```python
from build123d import *

# Parameters (mm, degrees)
SKETCH1_R           = 1.75
BOSS_EXTRUDE1_DEPTH = 1.6


with BuildPart() as part:
    # Sketch1 → Boss-Extrude1 (new body)
    with BuildSketch(Plane(origin=(0, 0, 0), x_dir=(1, 0, 0), z_dir=(0, 1, 0))):
        with BuildLine():
            Line((24.696313384, 21.403189927), (-19.414899465, 47.563680085))
            ThreePointArc((-19.414899465, 47.563680085), (-20.786874634, 49.384536896), (-20.482680557, 51.644028288))
            Line((-20.482680557, 51.644028288), (17.162414168, 116.847245007))
            ThreePointArc((17.162414168, 116.847245007), (19.546471274, 118.676596366), (22.525800971, 118.28436017))
            Line((22.525800971, 118.28436017), (70.987796177, 90.304814192))
            ThreePointArc((70.987796177, 90.304814192), (77.999004119, 90.304814192), (81.50460809, 96.376698381))
            Line((81.50460809, 96.376698381), (81.50460809, 182.02519482))
            ThreePointArc((81.50460809, 182.02519482), (80.873629228, 187.452491566), (79.01435205, 192.590270527))
            Line((79.01435205, 192.590270527), (69.144094326, 212.364639151))
            ThreePointArc((69.144094326, 212.364639151), (65.989183491, 217.196365343), (61.81193417, 221.177524531))
            Line((61.81193417, 221.177524531), (44.99314954, 233.854205885))
            Line((44.99314954, 233.854205885), (-23.199197227, 273.225075648))
            ThreePointArc((-23.199197227, 273.225075648), (-28.860512938, 273.225075648), (-31.691170793, 268.322232423))
            Line((-31.691170793, 268.322232423), (-31.691170793, 207.371759387))
            ThreePointArc((-31.691170793, 207.371759387), (-32.56985045, 205.250439044), (-34.691170793, 204.371759387))
            Line((-34.691170793, 204.371759387), (-106.595635326, 204.371759387))
            ThreePointArc((-106.595635326, 204.371759387), (-108.71695567, 205.250439044), (-109.595635326, 207.371759387))
            Line((-109.595635326, 207.371759387), (-109.595635326, 268.322232423))
            ThreePointArc((-109.595635326, 268.322232423), (-112.426293182, 273.225075648), (-118.087608892, 273.225075648))
            Line((-118.087608892, 273.225075648), (-186.279955659, 233.854205885))
            Line((-186.279955659, 233.854205885), (-204.21495553, 220.336208987))
            ThreePointArc((-204.21495553, 220.336208987), (-207.400637767, 217.300070339), (-209.806657286, 213.615266508))
            Line((-209.806657286, 213.615266508), (-217.247579174, 198.707901735))
            ThreePointArc((-217.247579174, 198.707901735), (-221.386722215, 187.270122423), (-222.791414209, 175.187815477))
            Line((-222.791414209, 175.187815477), (-222.791414209, 96.376698381))
            ThreePointArc((-222.791414209, 96.376698381), (-219.069332913, 89.929864467), (-211.625170321, 89.929864467))
            Line((-211.625170321, 89.929864467), (-163.512384372, 117.707794386))
            ThreePointArc((-163.512384372, 117.707794386), (-160.504762554, 118.10375531), (-158.098066116, 116.257032182))
            Line((-158.098066116, 116.257032182), (-120.496410943, 51.129054973))
            ThreePointArc((-120.496410943, 51.129054973), (-120.196709676, 48.852597838), (-121.594487155, 47.030978762))
            Line((-121.594487155, 47.030978762), (-165.983119503, 21.403189927))
            Line((-165.983119503, 21.403189927), (-174.676412504, 16.182853027))
            ThreePointArc((-174.676412504, 16.182853027), (-176.124776412, 13.818668342), (-175.016914475, 11.277060748))
            Line((-175.016914475, 11.277060748), (-168.860075369, 6.304549502))
            Line((-168.860075369, 6.304549502), (-141.286806119, 0))
            Line((-141.286806119, 0), (0, 0))
            Line((0, 0), (27.57326925, 6.304549502))
            Line((27.57326925, 6.304549502), (33.730108356, 11.277060748))
            ThreePointArc((33.730108356, 11.277060748), (34.837970293, 13.818668342), (33.389606385, 16.182853027))
            Line((33.389606385, 16.182853027), (24.696313384, 21.403189927))
        make_face()
        with Locations(Location((-123.091146174, 191.349343748, 0), (0, 0, 270))):
            Circle(SKETCH1_R, mode=Mode.SUBTRACT)
        with Locations(Location((-216.641081117, 98.036380822, 0), (0, 0, 270))):
            Circle(SKETCH1_R, mode=Mode.SUBTRACT)
        with Locations(Location((-18.645659945, 191.349343748, 0), (0, 0, 90))):
            Circle(SKETCH1_R, mode=Mode.SUBTRACT)
        with Locations(Location((74.914274997, 98.036380822, 0), (0, 0, 90))):
            Circle(SKETCH1_R, mode=Mode.SUBTRACT)
        with Locations(Location((-9.245725003, 21.35, 0), (0, 0, 270))):
            Circle(SKETCH1_R, mode=Mode.SUBTRACT)
        with Locations(Location((-132.441081117, 21.35, 0), (0, 0, 270))):
            Circle(SKETCH1_R, mode=Mode.SUBTRACT)
        with Locations(Location((-150.641414209, 135.049343748, 0), (0, 0, 270))):
            Circle(SKETCH1_R, mode=Mode.SUBTRACT)
        with Locations(Location((8.91460809, 135.049343748, 0), (0, 0, 270))):
            Circle(SKETCH1_R, mode=Mode.SUBTRACT)
        with Locations(Location((68.354340055, 202.349343748, 0), (0, 0, 270))):
            Circle(SKETCH1_R, mode=Mode.SUBTRACT)
        with Locations(Location((-11.691170793, 259.371759387, 0), (0, 0, 270))):
            Circle(SKETCH1_R, mode=Mode.SUBTRACT)
        with Locations(Location((-129.595635326, 259.371759387, 0), (0, 0, 270))):
            Circle(SKETCH1_R, mode=Mode.SUBTRACT)
        with Locations(Location((-209.641146174, 202.349343748, 0), (0, 0, 270))):
            Circle(SKETCH1_R, mode=Mode.SUBTRACT)
        Polygon((-31.555725003, 63.222149708), (-46.022445575, 49.606380822), (-95.264360544, 49.606380822), (-109.731081117, 63.222149708), (-109.731081117, 137.774232151), (-112.861146174, 137.774232151), (-112.861146174, 182.049343748), (-28.425659945, 182.049343748), (-28.425659945, 137.774232151), (-31.555725003, 137.774232151), align=None, mode=Mode.SUBTRACT)
    extrude(amount=BOSS_EXTRUDE1_DEPTH)


solid = part.part
```
Can you work these out from the model? Positions are in its coordinate system, mm. A direction names the side the tool comes from. Give positions to 0.01 mm unless a question says otherwise; leave off trailing zeros. Loops run counter-clockwise (first coordinate to the right, second up) from the corner with the lowest first, then second, coordinate; pieces in that order, holes last. Notation, with made-up numbers: M 36.5,60.5 L 68.5,60.5 A19 ccw 68.5,82.5 Z; hole C 78,-3.75 d4. An arc over 180 degrees is marked long. One line per question, with ' | ' between items. Start each with the question number.
Q1. If we section it at A-A (z = -227): Please give me the cut outline in (x, y).
Q2. For faces 4 (the flat face through (-143.478, 0.789, -34.396)), 5 (the cylindrical face through (66.041, 0.789, -217.134)), 6 (the flat face through (2.95, 0.79, -34.3)), 7 (the flat face through (-139.56, 0.79, -84.15)), which set-ups out of +Z, -Z, +X, -X, +Y, -Y let a thin tool reach every point of the face, with its end or its side?
Q3. If I drill on line 1 (X direction, y = 1.5, z = -191); line 2 (X direction, y = 1.5, z = -115); line 3 (Z direction, x = 10.5, y = 0.5), over which ranges is the centre line in solid material (lowest first)? Write a range as from..to.
Q4. For pin 1 Ø5.5 at (x, z) = (68.35, -202.35) entering from +Y; pin 2 Ø0.8 at (y, z) = (1, -247) entering from -X; pin 3 Ø0.8 at (x, y) = (-111, 1) entering from -Z, each with a flat end and sliding along its axis, tell me the tip position at first contact or that it passes through.
Q5. If we mould it in two halves opening along Z, with no side actions, what happens to faces 1 (the flat face through (-73, 1.6, -200)), 2 (the flat face through (-151.706, 0.789, -253.815)), 3 (the flat face through (46.4, 0.8, -104.5))? For each: +Z half, -Z half, draft (parallel to the pull), parting line (faces both ways), or undercut.
Q6. If we section it at B-B (y = 1.1): State how many separate pieces and enclosed holes the cut face has, plus the area to 3 significant figures.
Q7. If we section it at C-C (z = -67): Please give me the cut outline in (x, y), plus the area to 3 significant figures.
Computed:
1) outline: M -195.37,0 L -109.6,0 L -109.6,1.6 L -195.37,1.6 Z; M -31.69,0 L 54.09,0 L 54.09,1.6 L -31.69,1.6 Z
2) face 4: -X, +Y, -Y | face 5: -Z, +X, +Y, -Y | face 6: +X, +Y, -Y | face 7: +Y, -Y
3) line 1: x = -220.36..-124.81, -121.38..-20.36, -16.93..79.74 | line 2: x = -222.79..-168.2, -157.37..-109.73, -31.56..16.1, 28.21..81.5 | line 3: z = -253.77..-135.79, -134.31..-105.31, -29.82..-2.4
4) pin 1: stops at y = 1.6 | pin 2: stops at x = -164.2 | pin 3: stops at z = -272.47
5) face 1: draft | face 2: -Z half | face 3: undercut
6) separate pieces: 1 | enclosed holes: 13 | area: 44,000 mm²
7) outline: M -129.66,0 L -109.73,0 L -109.73,1.6 L -129.66,1.6 Z; M -31.56,0 L -11.62,0 L -11.62,1.6 L -31.56,1.6 Z | area: 63.8 mm²
